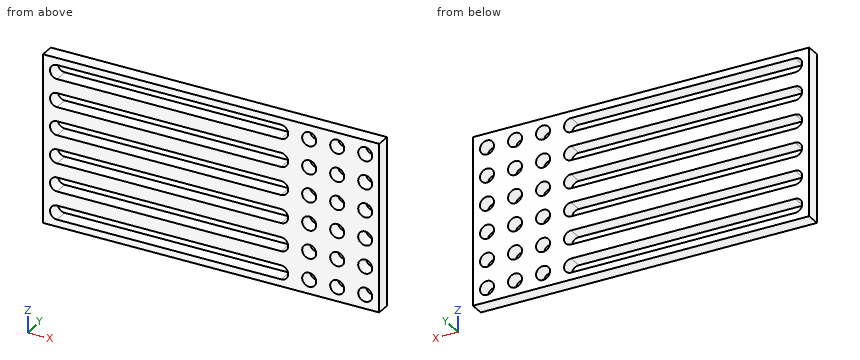
```python
from build123d import *

# Parameters (mm, degrees)
SKETCH1_W           = 152.4
SKETCH1_H           = 76.2
SKETCH1_R           = 3.175
BOSS_EXTRUDE1_DEPTH = 6.35


with BuildPart() as part:
    # Sketch1 → Boss-Extrude1 (new body)
    with BuildSketch(Plane(origin=(0, 0, 0), x_dir=(1, 0, 0), z_dir=(0, 1, 0))):
        Rectangle(SKETCH1_W, SKETCH1_H)
        with Locations(Location((44.45, 31.75, 0), (0, 0, 270))):
            Circle(SKETCH1_R, mode=Mode.SUBTRACT)
        with Locations(Location((57.15, 31.75, 0), (0, 0, 270))):
            Circle(SKETCH1_R, mode=Mode.SUBTRACT)
        with Locations(Location((69.85, 31.75, 0), (0, 0, 270))):
            Circle(SKETCH1_R, mode=Mode.SUBTRACT)
        with Locations(Location((44.45, 19.05, 0), (0, 0, 270))):
            Circle(SKETCH1_R, mode=Mode.SUBTRACT)
        with Locations(Location((57.15, 19.05, 0), (0, 0, 270))):
            Circle(SKETCH1_R, mode=Mode.SUBTRACT)
        with Locations(Location((69.85, 19.05, 0), (0, 0, 270))):
            Circle(SKETCH1_R, mode=Mode.SUBTRACT)
        with Locations(Location((44.45, 6.35, 0), (0, 0, 270))):
            Circle(SKETCH1_R, mode=Mode.SUBTRACT)
        with Locations(Location((57.15, 6.35, 0), (0, 0, 270))):
            Circle(SKETCH1_R, mode=Mode.SUBTRACT)
        with Locations(Location((69.85, 6.35, 0), (0, 0, 270))):
            Circle(SKETCH1_R, mode=Mode.SUBTRACT)
        with Locations(Location((44.45, -6.35, 0), (0, 0, 270))):
            Circle(SKETCH1_R, mode=Mode.SUBTRACT)
        with Locations(Location((57.15, -6.35, 0), (0, 0, 270))):
            Circle(SKETCH1_R, mode=Mode.SUBTRACT)
        with Locations(Location((69.85, -6.35, 0), (0, 0, 270))):
            Circle(SKETCH1_R, mode=Mode.SUBTRACT)
        with Locations(Location((44.45, -19.05, 0), (0, 0, 270))):
            Circle(SKETCH1_R, mode=Mode.SUBTRACT)
        with Locations(Location((57.15, -19.05, 0), (0, 0, 270))):
            Circle(SKETCH1_R, mode=Mode.SUBTRACT)
        with Locations(Location((69.85, -19.05, 0), (0, 0, 270))):
            Circle(SKETCH1_R, mode=Mode.SUBTRACT)
        with Locations(Location((44.45, -31.75, 0), (0, 0, 270))):
            Circle(SKETCH1_R, mode=Mode.SUBTRACT)
        with Locations(Location((57.15, -31.75, 0), (0, 0, 270))):
            Circle(SKETCH1_R, mode=Mode.SUBTRACT)
        with Locations(Location((69.85, -31.75, 0), (0, 0, 270))):
            Circle(SKETCH1_R, mode=Mode.SUBTRACT)
        with BuildLine():
            Line((-69.85, 34.925), (31.75, 34.925))
            ThreePointArc((31.75, 34.925), (34.925, 31.75), (31.75, 28.575))
            Line((31.75, 28.575), (-69.85, 28.575))
            ThreePointArc((-69.85, 28.575), (-73.025, 31.75), (-69.85, 34.925))
        make_face(mode=Mode.SUBTRACT)
        with BuildLine():
            Line((31.75, 15.875), (-69.85, 15.875))
            ThreePointArc((-69.85, 15.875), (-73.025, 19.05), (-69.85, 22.225))
            Line((-69.85, 22.225), (31.75, 22.225))
            ThreePointArc((31.75, 22.225), (34.925, 19.05), (31.75, 15.875))
        make_face(mode=Mode.SUBTRACT)
        with BuildLine():
            Line((31.75, 3.175), (-69.85, 3.175))
            ThreePointArc((-69.85, 3.175), (-73.025, 6.35), (-69.85, 9.525))
            Line((-69.85, 9.525), (31.75, 9.525))
            ThreePointArc((31.75, 9.525), (34.925, 6.35), (31.75, 3.175))
        make_face(mode=Mode.SUBTRACT)
        with BuildLine():
            Line((31.75, -9.525), (-69.85, -9.525))
            ThreePointArc((-69.85, -9.525), (-73.025, -6.35), (-69.85, -3.175))
            Line((-69.85, -3.175), (31.75, -3.175))
            ThreePointArc((31.75, -3.175), (34.925, -6.35), (31.75, -9.525))
        make_face(mode=Mode.SUBTRACT)
        with BuildLine():
            Line((31.75, -22.225), (-69.85, -22.225))
            ThreePointArc((-69.85, -22.225), (-73.025, -19.05), (-69.85, -15.875))
            Line((-69.85, -15.875), (31.75, -15.875))
            ThreePointArc((31.75, -15.875), (34.925, -19.05), (31.75, -22.225))
        make_face(mode=Mode.SUBTRACT)
        with BuildLine():
            Line((31.75, -34.925), (-69.85, -34.925))
            ThreePointArc((-69.85, -34.925), (-73.025, -31.75), (-69.85, -28.575))
            Line((-69.85, -28.575), (31.75, -28.575))
            ThreePointArc((31.75, -28.575), (34.925, -31.75), (31.75, -34.925))
        make_face(mode=Mode.SUBTRACT)
    extrude(amount=BOSS_EXTRUDE1_DEPTH)


solid = part.part
```
Build history of the part. All positions in model axes, mm. Round coordinates to 2 decimals unless told otherwise and drop trailing zeros. Write each loop counter-clockwise with the first axis right and the second up, starting at its lowest first coordinate (ties: lowest second). Pieces come first, ordered by that corner, then holes.
1) Band-saw the part on D-D, the plane y = 2.75. Give the number of separate pieces and of enclosed holes in the cut face, and give its area (3 significant figures).
2) Band-saw the part on B-B, the plane z = -19.05. List the corners of the cut face in (x, y) (3 decimals).
3) Band-saw the part on A-A, the plane x = 57.15. List the corners of the cut face in (y, z) (3 decimals).
4) Drill centre lines: probe 1 along X at (y, z) = (4.25, -19.05) (3 decimals); probe 2 along X at (y, z) = (4, -5). Where is each one in solid material? Low to high.
5) Band-saw the part on C-C, the plane z = 8. List the corners of the cut face in (x, y).
Ans:
1. separate pieces: 1
1. enclosed holes: 24
1. area: 6,980 mm2
2. outline: (-76.2, 0) - (-73.025, 0) - (-73.025, 6.35) - (-76.2, 6.35) - close; (34.925, 0) - (41.275, 0) - (41.275, 6.35) - (34.925, 6.35) - close; (47.625, 0) - (53.975, 0) - (53.975, 6.35) - (47.625, 6.35) - close; (60.325, 0) - (66.675, 0) - (66.675, 6.35) - (60.325, 6.35) - close; (73.025, 0) - (76.2, 0) - (76.2, 6.35) - (73.025, 6.35) - close
3. outline: (0, -38.1) - (6.35, -38.1) - (6.35, -34.925) - (0, -34.925) - close; (0, -28.575) - (6.35, -28.575) - (6.35, -22.225) - (0, -22.225) - close; (0, -15.875) - (6.35, -15.875) - (6.35, -9.525) - (0, -9.525) - close; (0, -3.175) - (6.35, -3.175) - (6.35, 3.175) - (0, 3.175) - close; (0, 9.525) - (6.35, 9.525) - (6.35, 15.875) - (0, 15.875) - close; (0, 22.225) - (6.35, 22.225) - (6.35, 28.575) - (0, 28.575) - close; (0, 34.925) - (6.35, 34.925) - (6.35, 38.1) - (0, 38.1) - close
4. probe 1: x = -76.2 to -73.025, 34.925 to 41.275, 47.625 to 53.975, 60.325 to 66.675, 73.025 to 76.2
4. probe 2: x = -76.2 to -72.72, 34.62 to 41.58, 47.32 to 54.28, 60.02 to 66.98, 72.72 to 76.2
5. outline: (-76.2, 0) - (-72.56, 0) - (-72.56, 6.35) - (-76.2, 6.35) - close; (34.46, 0) - (41.74, 0) - (41.74, 6.35) - (34.46, 6.35) - close; (47.16, 0) - (54.44, 0) - (54.44, 6.35) - (47.16, 6.35) - close; (59.86, 0) - (67.14, 0) - (67.14, 6.35) - (59.86, 6.35) - close; (72.56, 0) - (76.2, 0) - (76.2, 6.35) - (72.56, 6.35) - close
